Autodesk Inventor part; units mm, degrees
ref_plane "YZ Plane" through (0, 0, 0) normal (1, 0, 0) x (0, 1, 0)
ref_plane "XZ Plane" through (0, 0, 0) normal (0, 1, 0) x (-1, 0, 0)
ref_plane "XY Plane" through (0, 0, 0) normal (0, 0, 1) x (1, 0, 0)
sketch "Boceto1" plane through (0, 0, 0) normal (0, 1, 0) x (-1, 0, 0)
  line L0 (0, 0) -> (30, 0)
  line L1 (30, 0) -> (30, -10)
  line L2 (30, -10) -> (30, -10)
  line L3 (30, -10) -> (30, -22)
  line L4 (30, -22) -> (30, -22)
  line L5 (30, -22) -> (30, -32)
  line L6 (30, -32) -> (0, -32)
  line L7 (0, -32) -> (0, -22)
  line L8 (0, -22) -> (0, -22)
  line L9 (0, -22) -> (0, -10)
  line L10 (0, -10) -> (0, -10)
  line L11 (0, 0) -> (0, -10)
  line L12 (15, -32) -> (15, -22)
  circle A0 centre (15, -22) radius 4.25
  dimension "d0" = 30
  dimension "d1" = 10
  dimension "d2" = 0
  dimension "d3" = 12
  dimension "d4" = 10
  dimension "d5" = 10
  dimension "d6" = 0
  dimension "d10" = 8.5
extrude "Extrusión2" add sketch "Boceto1" along normal blind 3
fillet "Empalme1" radius 0.5 2 edges at (-10.75, 3, -22) (-10.75, 0, -22)
sketch "Sketch4" plane through (0, 0, 0) normal (0, -1, 0) x (1, 0, 0)
  line L0 (-30, 0) -> (-27.5, 0)
  line L1 (-30, 0) -> (0, 0)
  line L2 (-27.5, 0) -> (-27.5, -2.5)
  line L3 (0, 0) -> (-2.5, 0)
  line L4 (-2.5, 0) -> (-2.5, -2.5)
  line L5 (0, -32) -> (-2.5, -32)
  line L6 (0, -32) -> (-30, -32)
  line L7 (-2.5, -32) -> (-2.5, -29.5)
  line L8 (-30, -32) -> (-27.5, -32)
  line L9 (-27.5, -32) -> (-27.5, -29.5)
  circle A0 centre (-27.5, -2.5) radius 1.5
  circle A1 centre (-2.5, -2.5) radius 1.5
  circle A2 centre (-2.5, -29.5) radius 1.5
  circle A3 centre (-27.5, -29.5) radius 1.5
  dimension "d20" = 2.5
  dimension "d21" = 2.5
  dimension "d22" = 2.5
  dimension "d23" = 2.5
  dimension "d24" = 2.5
  dimension "d25" = 2.5
  dimension "d26" = 2.5
  dimension "d27" = 2.5
  dimension "d28" = 3
  dimension "d29" = 3
  dimension "d30" = 3
  dimension "d31" = 3
extrude "Extrusion4" cut sketch "Sketch4" against normal through all
properties part number "core_case"
Source: CAD feature listing. Evaluate the final solid. Frame: model axes, mm. Give positions to 0.01 mm unless a question says otherwise; leave off trailing zeros. Order: outer loops, then holes, each group sorted by start corner. A loop starts at its lowest first (then second) coordinate and runs counter-clockwise, first axis right, second up. Notation, with made-up numbers: (-9, -32.5) -> (28, -32.5) arc R28 cw to (28, 4.5) -> close; hole circle Ø11 at (23, 75.5). An arc over 180 degrees is marked (long way). Use a Markdown table: item, result.
1) Section query D-D, the plane x = -15. Return the cut outline in (y, z), then the cut area to 3 significant figures.
Answer list:
| item | result |
|---|---|
| outline | (0, -32) -> (3, -32) -> (3, -26.75) arc R0.5 ccw to (2.5, -26.25) -> (0.5, -26.25) arc R0.5 ccw to (0, -26.75) -> close; (0, -17.25) arc R0.5 ccw to (0.5, -17.75) -> (2.5, -17.75) arc R0.5 ccw to (3, -17.25) -> (3, 0) -> (0, 0) -> close |
| area | 70.3 mm² |
2) Mould query, pull axis X, two halves, no side actions, for faces 1 (the flat face through (-30, 1, -16)), 2 (the cylindrical face through (-1.694, 1.479, -1.235)), 3 (the flat face through (-15, 1, -32)). Classes: +X half, -X half, draft (parallel to the pull), parting line (faces both ways), or undercut.
Answer list:
| item | result |
|---|---|
| face 1 | -X half |
| face 2 | undercut |
| face 3 | draft |
3) Section query A-A, the plane z = -22. Return the cut outline in (x, y).
Answer list:
| item | result |
|---|---|
| outline | (-30, 0) -> (-19.75, 0) arc R0.5 ccw to (-19.25, 0.5) -> (-19.25, 2.5) arc R0.5 ccw to (-19.75, 3) -> (-30, 3) -> close; (-10.75, 0.5) arc R0.5 ccw to (-10.25, 0) -> (0, 0) -> (0, 3) -> (-10.25, 3) arc R0.5 ccw to (-10.75, 2.5) -> close |
4) Section query C-C, the plane y = 1.4. Return the cut outline in (x, z).
Answer list:
| item | result |
|---|---|
| outline | (-30, -32) -> (0, -32) -> (0, 0) -> (-30, 0) -> close; hole circle Ø3 at (-27.5, -29.5); hole circle Ø3 at (-27.5, -2.5); hole circle Ø8.5 at (-15, -22); hole circle Ø3 at (-2.5, -29.5); hole circle Ø3 at (-2.5, -2.5) |
5) Ray query, line 1 along Z through (x, y) = (-27.5, 1.2); line 2 along X through (y, z) = (1.85, -2.5); line 3 along X through (y, z) = (1.95, -22). Return the intervals inside material, ascending. Write a range as [from, to].
Answer list:
| item | result |
|---|---|
| line 1 | [-32, -31], [-28, -4], [-1, 0] |
| line 2 | [-30, -29], [-26, -4], [-1, 0] |
| line 3 | [-30, -19.25], [-10.75, 0] |
6) Contact query for a flat-ended pin moving along its axis: P1, Ø4, axis at x = -15.5, z = -22.5, coming from the -Y side. Output: stop coordinate, or through.
Answer list:
| item | result |
|---|---|
| P1 | through |
7) Section query B-B, the plane x = -2.5. Return the cut outline in (y, z).
Answer list:
| item | result |
|---|---|
| outline | (0, -32) -> (3, -32) -> (3, -31) -> (0, -31) -> close; (0, -28) -> (3, -28) -> (3, -4) -> (0, -4) -> close; (0, -1) -> (3, -1) -> (3, 0) -> (0, 0) -> close |
